Could you check a few things on this model? Use its own coordinates, in mm. A direction names the side the tool comes from. Coordinates: 2 decimals unless noted, no trailing zeros. One line per question, with ' | ' between items.
from build123d import *

# Parameters (mm, degrees)
CUT_EXTRUDE1_DEPTH      = 60
CUT_EXTRUDE1_DEPTH_BACK = 60
SKETCH2_R               = 10


with BuildPart() as part:
    # Sketch1 → Revolve1 (revolve)
    with BuildSketch(Plane.XY, mode=Mode.PRIVATE) as revolve1_sk:
        with BuildLine():
            Line((-50.213491879, 0), (-50.213491879, 60))
            Line((-50.213491879, 60), (-43.142539091, 60))
            Line((-43.142539091, 60), (-43.142539091, 65))
            Line((-43.142539091, 65), (-50.213491879, 65))
            Line((-50.213491879, 65), (-50.213491879, 70))
            Line((-50.213491879, 70), (-43.142539091, 70))
            Line((-43.142539091, 70), (-43.142539091, 75))
            Line((-43.142539091, 75), (-50.213491879, 75))
            Line((-50.213491879, 75), (-50.213491879, 80))
            Line((-50.213491879, 80), (-43.142539091, 80))
            Line((-43.142539091, 80), (-43.142539091, 85))
            Line((-43.142539091, 85), (-50.213491879, 85))
            Line((-50.213491879, 85), (-50.213491879, 100))
            Line((-50.213491879, 100), (-29.758235601, 100))
            ThreePointArc((-29.758235601, 100), (-27.613235974, 94.821512811), (-22.434748785, 92.676513184))
            Line((-22.434748785, 92.676513184), (-11.323251547, 91.161309016))
            Line((-11.323251547, 91.161309016), (0, 91.161309016))
            Line((0, 91.161309016), (0, 0))
            Line((0, 0), (-50.213491879, 0))
        make_face()
    revolve(revolve1_sk.sketch.rotate(Axis((0, 116.04188361, 0), (0, -1, 0)), 270), axis=Axis((0, 116.04188361, 0), (0, -1, 0)))

    # Shell1: read off the stored shape, not the designer's step
    # Shell1 outline → Shell1 (revolve, cut)
    with BuildSketch(Plane.XY):
        with BuildLine():
            Line((12.001929251, 81.161309016), (0, 81.161309016))
            Line((0, 81.161309016), (0, 0))
            Line((0, 0), (40.213491879, 0))
            Line((40.213491879, 0), (40.213491879, 50))
            Line((40.213491879, 50), (33.142539091, 50))
            Line((33.142539091, 50), (33.142539091, 86.382128573))
            ThreePointArc((33.142539091, 86.382128573), (28.486928042, 83.768107883), (23.256399997, 82.696009572))
            Line((23.256399997, 82.696009572), (12.001929251, 81.161309016))
        make_face()
    revolve(axis=Axis((0, 0, 0), (0, 1, 0)), mode=Mode.SUBTRACT)

    # Sketch2 → Cut-Extrude1 (cut, two sides: drawn at the far end of the back side and taken through both)
    with BuildSketch(Plane(origin=(0, 0, 0), x_dir=(0, 0, -1), z_dir=(1, 0, 0)).offset(-CUT_EXTRUDE1_DEPTH_BACK)):
        with Locations(Location((-0.200994326, 38.878313976, 0), (0, 0, 180))):
            Circle(SKETCH2_R)
        with BuildLine():
            Line((-33.49905429, 0), (33.097065639, 0))
            ThreePointArc((33.097065639, 0), (-0.200994326, 19.719751163), (-33.49905429, 0))
        make_face()
    extrude(amount=CUT_EXTRUDE1_DEPTH + CUT_EXTRUDE1_DEPTH_BACK, mode=Mode.SUBTRACT)


solid = part.part
1) On a 3-axis mill with a long thin cutter (end or side, diameter ignored), from which of +Z, -Z, +X, -X, +Y, -Y can I reach the whole of each face in a straight line? I mean faces 5 (the face through (15.3, 68.4, 29.4)), 6 (the face through (22, 100, 22)), 7 (the face through (-37.4, 65, -22.1)). Say none if no direction works.
Data:
face 5: -Y | face 6: +Z, -Z, +X, -X, +Y | face 7: none
2) If we section it at B-B on z = 0: Give the number of separate pieces and of enclosed holes in the cut face, and give its area (3 significant figures).
Data:
separate pieces: 3 | enclosed holes: 0 | area: 2,410 mm²
3) I'm going to push flat-ended pins straight in: pin 1 Ø2 at (y, z) = (39, -12.5) entering from -X; pin 2 Ø5 at (x, y) = (-13, 32) entering from +Z; pin 3 Ø8 at (y, z) = (41, -8) entering from +X; pin 4 Ø12 at (y, z) = (38.88, 0.2) entering from -X. Where does each tip first touch, or does it pass through?
Data:
pin 1: x = -48.88 | pin 2: z = 49.1 | pin 3: x = 49.62 | pin 4: through
4) We'd pull the mould along Z, two halves only. Please class faces 1 (the face through (-42.775, 72.535, -5.616)), 2 (the face through (44.48, 48.64, -1.97)), 3 (the face through (0, 91.161, 0)), 4 (the face through (-37.4, 85, -22.1)): pulls with the +Z half, pulls with the -Z half, needs draft (parallel to the pull), parting line crosses it, or undercut.
Data:
face 1: parting line crosses it | face 2: undercut | face 3: undercut | face 4: needs draft
5) I need wall thicknesses on line 1 along Y through (x, z) = (22.5, 39.5); line 2 along X through (y, z) = (22, 0); line 3 along X through (y, z) = (76, 0). Which ranges of each line are inside material? Lowest first, please. Write a range as from..to.
Data:
line 1: 0..60, 65..70, 75..80, 85..100 | line 2: -50.21..-40.21, 40.21..50.21 | line 3: -50.21..-33.14, 33.14..50.21
